Geometry: see drawing. Coordinates: mm, zero at the bounding-box minimum. Coordinates: 2 decimals unless noted, no trailing zeros. Order: outer loops, then holes, each group sorted by start corner. A loop starts at its lowest first (then second) coordinate and runs counter-clockwise, first axis right, second up.
Item 1: Contact query for flat-ended pins moving along their axis: P1, Ø1.5, axis at x = 95, y = 22.5, coming from the +Z side; P2, Ø5, axis at x = 76.2, y = 76.2, coming from the +Z side; P3, Ø4, axis at x = 106, z = 90, coming from the +Y side; P4, Ø3, axis at x = 107.5, y = 92.5, coming from the -Z side. Output: stop coordinate, or through.
Item 2: Section C-C on z = 59. Return the cut outline in (x, y) (3 decimals), then the cut area to 3 significant figures.
Item 3: Section A-A on y = 76.2. Return the cut outline in (x, z) (3 decimals).
Item 4: Ray query, line 1 (Y direction, x = 76.2, z = 63) (3 decimals); line 2 (X direction, y = 76, z = 58); line 3 (Y direction, x = 77, z = 33). Return the intervals inside material, ascending.
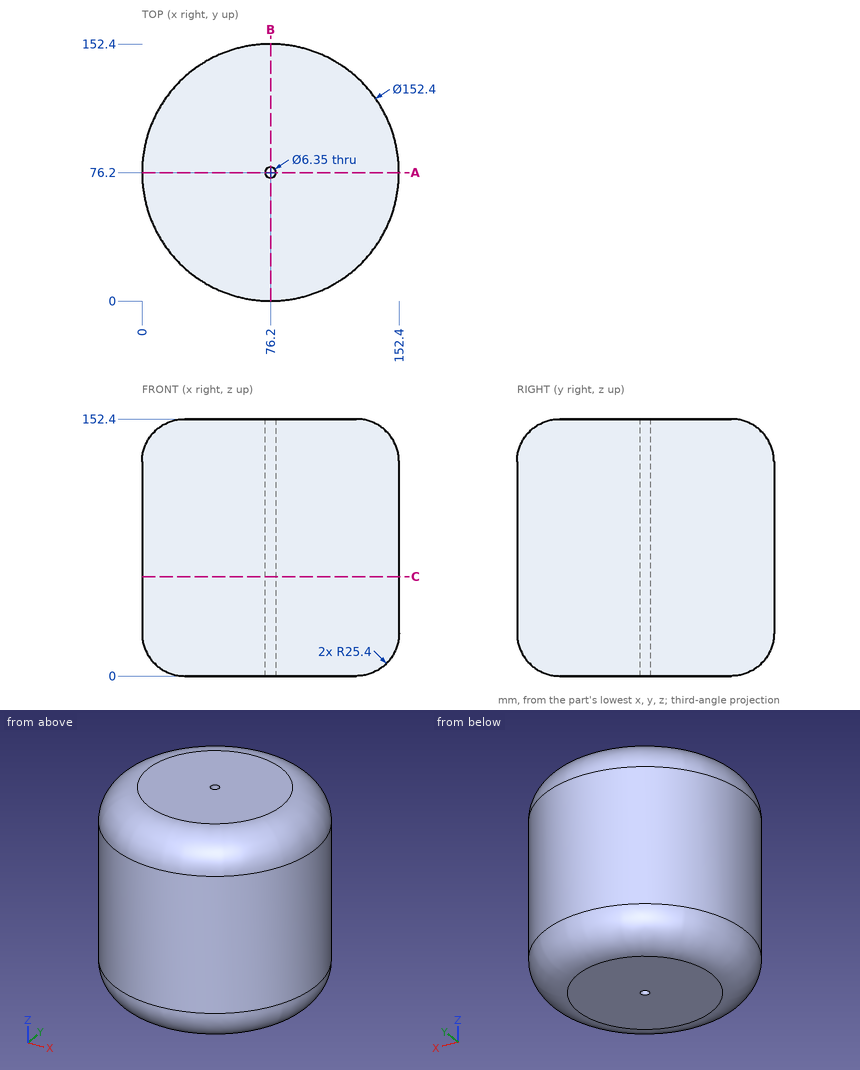
Answer list:
1. P1: stops at z = 151.83
1. P2: passes through
1. P3: stops at y = 147.15
1. P4: stops at z = 0
2. outline: circle Ø152.4 at (76.2, 76.2); hole circle Ø6.35 at (76.2, 76.2)
2. area: 18,200 mm2
3. outline: (0, 25.4) arc R25.4 ccw to (25.4, 0) - (73.025, 0) - (73.025, 152.4) - (25.4, 152.4) arc R25.4 ccw to (0, 127) - close; (79.375, 0) - (127, 0) arc R25.4 ccw to (152.4, 25.4) - (152.4, 127) arc R25.4 ccw to (127, 152.4) - (79.375, 152.4) - close
4. line 1: y = 0 to 73.025, 79.375 to 152.4
4. line 2: x = 0 to 73.03, 79.37 to 152.4
4. line 3: y = 0 to 73.13, 79.27 to 152.4
